Autodesk Inventor part; units mm, degrees
ref_plane "Work Plane1" through (10, 0, 0) normal (0, 0, 1) x (1, 0, 0)
ref_plane "YZ Plane" through (0, 0, 0) normal (1, 0, 0) x (0, 1, 0)
ref_plane "XZ Plane" through (0, 0, 0) normal (0, 1, 0) x (-1, 0, 0)
sketch "Skizze1" plane through (0, 0, 0) normal (0, 0, 1) x (1, 0, 0)
  line L0 (0, 0) -> (17.5, 0)
  line L1 (20, 0.866) -> (20, 1.5)
  line L2 (20, 1.5) -> (0, 1.5)
  line L3 (20, 0.866) -> (18, 0.866)
  line L4 (18, 0.866) -> (17.5, 0)
  line L5 (0, -0.3) -> (0, 1.8)
  line L6 (0, 1.5) -> (0, 0)
  dimension "d0" = 2
  dimension "d1" = 60
  dimension "d2" = 3
  dimension "d3" = 1.7321
  dimension "d5" = 20
revolve "Körper" add sketch "Skizze1" angle 360 about axis through (0, 0, 0) along (1, 0, 0)
sketch "Skizze2" plane through (20, 0, 0) normal (1, 0, 0) x (0, 1, 0)
  circle A0 centre (0, 0) radius 0.866
  line L0 (-0.433, 0.75) -> (0.433, 0.75)
  line L1 (0.433, 0.75) -> (0.866, 0)
  line L2 (0.866, 0) -> (0.433, -0.75)
  line L3 (0.433, -0.75) -> (-0.433, -0.75)
  line L4 (-0.433, -0.75) -> (-0.866, 0)
  line L5 (-0.866, 0) -> (-0.433, 0.75)
  point P0 (0, 0)
  point P1 (0, 0)
extrude "Loch" add sketch "Skizze2" against normal up to next contours L1 A0 | A0 L2 | L0 A0 | A0 L3 | L5 A0 | A0 L4
thread "Gewinde"
chamfer "Fase1" distance 1.5 angle 45 1 edges at (0, -1.5, 0) measured on face at (13.3333, 1.4951, -0.1207)
chamfer "Fase2" distance 0.3067 angle 45 1 edges at (20, -1.5, 0) measured on face at (13.8332, 1.4806, -0.2406)
ref_plane "Work Plane1" through (10, 0, 0) normal (0, 0, 1) x (1, 0, 0)
equation "\"d0\" = INTI"
equation "\"d2\" = NND"
equation "\"d3\" = 1.1547 * SW"
equation "\"d5\" = NLG"
equation "\"d12\" = NLG"
equation "\"d9\" = FAWI"
equation "\"d10\" = -0.5 * GD1 + 0.5 * NND"
equation "\"d11\" = FAWI"
equation "\"d35\" = -0.5 * GD1 + 0.5 * NND"
equation "\"NND\" = 3"
equation "\"NLG\" = 20"
equation "\"INTI\" = 2"
equation "\"FAWI\" = 45deg"
equation "\"SW\" = 1.5"
equation "\"GD1\" = THREADDIA - 1.2269 * PTC"
equation "\"FAWI1\" = 45deg"
equation "\"SPD\" = 0.00001"
equation "\"GUL\" = 0.61345 * PTC"
equation "\"TOA\" = 30deg"
equation "\"THREADDIA\" = 3"
equation "\"PTC\" = 0.5"
equation "\"GAL\" = 0.61345 * PTC"
equation "\"E0\" = 1.155 * SW"
properties part number "DIN 914 - M3 x 20" material "Stahl, weich"
Verification items for the finished model (mm, model axes). Coordinates: 2 decimals unless noted, no trailing zeros. Order: outer loops, then holes, each group sorted by start corner. A loop starts at its lowest first (then second) coordinate and runs counter-clockwise, first axis right, second up. Notation, with made-up numbers: (22, 66.25) -> (28, 66.25) arc R17 cw to (28, 87.25) -> close; hole circle Ø6 at (4, 16.25). An arc over 180 degrees is marked (long way). Use CSV: the item, a comma, the result in double quotes. Start each with the question number.
Q1. Thickness scan on line 1 along Z through (x, y) = (2, 0.1); line 2 along Y through (x, z) = (11, -1.3). Record the ranges inside material, lowest first.
Q2. Section check A-A, the plane x = 2.5. Record the cut outline in (y, z).
Q3. Draft check along Z on faces 1 (the flat face through (19, 0, 0.75)), 2 (the flat face through (20, 0, -1)), 3 (the flat face through (19, 0, -0.75)), 4 (the conical face through (0, 0, 0)). Enter one of: +Z half, -Z half, draft (parallel to the pull), parting line (faces both ways), or undercut.
Q4. Depth check by flat-ended pin: P1, Ø1, axis at y = 0.5, z = 0, coming from the +X side. Enter the tip coordinate at first touch or a pass-through.
Returned:
1,line 1,"z = -1.5 to 1.5"
1,line 2,"y = -0.75 to 0.75"
2,outline,"circle Ø3 at (0, 0)"
3,face 1,"undercut"
3,face 2,"draft"
3,face 3,"undercut"
3,face 4,"parting line"
4,P1,"stops at x = 20"
